```python
from build123d import *

# Parameters (mm, degrees)
F0_R          = 44.45
F0_R_2        = 41.275
F1_DEPTH      = 63.5
F1_DEPTH_BACK = 63.5
F3_DEPTH      = 57.912
F5_DEPTH      = 91.694
F7_DEPTH      = 40.132


with BuildPart() as f1:
    # F0 (on Right) → F1 (new body, two sides)
    with BuildSketch(Plane.YZ) as f1_sk:
        Circle(F0_R)
        Circle(F0_R_2, mode=Mode.SUBTRACT)
    extrude(amount=F1_DEPTH)
    extrude(f1_sk.sketch, amount=-F1_DEPTH_BACK)

    # F2 (on Front) → F3 (cut)
    with BuildSketch(Plane.XZ):
        Polygon((-35.56, 0), (0, 0), (35.56, 0), (11.43, 38.338508), (0, 38.338508), (-11.43, 38.338508), align=None)
    extrude(amount=F3_DEPTH, mode=Mode.SUBTRACT)

    # F4 (on Top) → F5 (cut)
    with BuildSketch(Plane.XY):
        Polygon((-11.43, -23.685547), (0, -23.685547), (11.43, -23.685547), (11.43, 27.390007), (-11.43, 27.390007), align=None)
    extrude(amount=F5_DEPTH, mode=Mode.SUBTRACT)

    # F6 (on Front) → F7 (cut)
    with BuildSketch(Plane.XZ):
        Polygon((-11.43, 0), (0, 0), (11.43, 0), (11.43, 35.2511), (0, 35.2511), (-11.43, 35.2511), align=None)
    extrude(amount=-F7_DEPTH, mode=Mode.SUBTRACT)


solid = f1.part
```
The listing builds one solid part. Answer for the finished solid, in the listing's coordinates (mm). Give positions to 0.01 mm unless a question says otherwise; leave off trailing zeros. Order: outer loops, then holes, each group sorted by start corner. A loop starts at its lowest first (then second) coordinate and runs counter-clockwise, first axis right, second up.
1) Given P1, Ø10, axis at x = 10, y = -33, coming from the +Z side; P2, Ø6, axis at x = -37.5, y = -35, coming from the +Z side; P3, Ø1.5, axis at y = 32.5, z = -21, coming from the +X side; P4, Ø10, axis at x = -11.5, y = 23, coming from the -Z side, each flat-ended and moving along its own axis, determine where each tip first touches the part or whether it passes through.
Reported:
P1: stops at z = -16.11
P2: stops at z = 30.85
P3: passes through
P4: stops at z = -40.64
2) Find section A-A on y = 0. Write down the section's boundary in (x, z) (3 decimals).
Reported:
outline: (-63.5, -44.45) - (63.5, -44.45) - (63.5, -41.275) - (-63.5, -41.275) - close; (-63.5, 41.275) - (-11.43, 41.275) - (-11.43, 44.45) - (-63.5, 44.45) - close; (11.43, 41.275) - (63.5, 41.275) - (63.5, 44.45) - (11.43, 44.45) - close
3) Find section D-D on y = -29.5. Write down the section's boundary in (x, z).
Reported:
outline: (-63.5, -33.25) - (63.5, -33.25) - (63.5, -28.87) - (-63.5, -28.87) - close; (-63.5, 28.87) - (-17.39, 28.87) - (-14.63, 33.25) - (-63.5, 33.25) - close; (14.63, 33.25) - (17.39, 28.87) - (63.5, 28.87) - (63.5, 33.25) - close
4) Find section C-C on x = -52.5. Write down the section's boundary in (y, z) (3 decimals), then the cut area to 3 significant figures.
Reported:
outline: circle Ø88.9 at (0, 0); hole circle Ø82.55 at (0, 0)
area: 855 mm2
5) Consider line 1 along Y through (x, z) = (-37, 0) (3 decimals); line 2 along Z through (x, y) = (-55, -35.5). Determine where each line is inside the solid, lowest interval first.
Reported:
line 1: y = -44.45 to -41.275, 41.275 to 44.45
line 2: z = -26.75 to -21.06, 21.06 to 26.75
6) Find section B-B on z = -18. Write down the section's boundary in (x, y), then the cut area to 3 significant figures.
Reported:
outline: (-63.5, -40.64) - (63.5, -40.64) - (63.5, -37.14) - (-63.5, -37.14) - close; (-63.5, 37.14) - (63.5, 37.14) - (63.5, 40.64) - (-63.5, 40.64) - close
area: 889 mm2
7) Determine the mould class of faces 1 (the face through (0, -43, 0)), 2 (the face through (0.889, 38.128, -15.809)), 3 (the face through (0, 40.132, 14)), 4 (the face through (0.889, 41.061, -17.025)) for opening direction Y: pulls with the +Y half, pulls with the -Y half, needs draft (parallel to the pull), parting line crosses it, or undercut.
Reported:
face 1: needs draft
face 2: undercut
face 3: pulls with the -Y half
face 4: parting line crosses it
